```python
from build123d import *

# Parameters (mm, degrees)
SKETCH1_R           = 1.27
BOSS_EXTRUDE1_DEPTH = 0.4
SKETCH2_W           = 11.275942915
SKETCH2_H           = 6.002616378
BOSS_EXTRUDE2_DEPTH = 2.4


with BuildPart() as part:
    # Sketch1 → Boss-Extrude1 (new body)
    with BuildSketch(Plane(origin=(0, 0, 0), x_dir=(1, 0, 0), z_dir=(0, 1, 0))):
        with BuildLine():
            Line((13.97, -10.16), (-13.97, -10.16))
            ThreePointArc((-13.97, -10.16), (-15.766051224, -9.416051224), (-16.51, -7.62))
            Line((-16.51, -7.62), (-16.51, 7.62))
            ThreePointArc((-16.51, 7.62), (-15.766051224, 9.416051224), (-13.97, 10.16))
            Line((-13.97, 10.16), (13.97, 10.16))
            ThreePointArc((13.97, 10.16), (15.766051224, 9.416051224), (16.51, 7.62))
            Line((16.51, 7.62), (16.51, -7.62))
            ThreePointArc((16.51, -7.62), (15.766051224, -9.416051224), (13.97, -10.16))
        make_face()
        with Locations(Location((-13.97, 7.62, 0), (0, 0, 270))):
            Circle(SKETCH1_R, mode=Mode.SUBTRACT)
        with Locations(Location((13.97, 7.62, 0), (0, 0, 270))):
            Circle(SKETCH1_R, mode=Mode.SUBTRACT)
        with Locations(Location((13.97, -7.62, 0), (0, 0, 270))):
            Circle(SKETCH1_R, mode=Mode.SUBTRACT)
        with Locations(Location((-13.97, -7.62, 0), (0, 0, 270))):
            Circle(SKETCH1_R, mode=Mode.SUBTRACT)
    extrude(amount=BOSS_EXTRUDE1_DEPTH)

    # Sketch2 → Boss-Extrude2 (add)
    with BuildSketch(Plane(origin=(0, 0.4, 0), x_dir=(1, 0, 0), z_dir=(0, 1, 0))):
        with Locations((-5.637971457, 0)):
            Rectangle(SKETCH2_W, SKETCH2_H)
    extrude(amount=BOSS_EXTRUDE2_DEPTH)


solid = part.part
```
Part model, mm, in its own coordinate system. A direction names the side the tool comes from. Give positions to 0.01 mm unless a question says otherwise; leave off trailing zeros. Write each loop counter-clockwise with the first axis right and the second up, starting at its lowest first coordinate (ties: lowest second). Pieces come first, ordered by that corner, then holes. Notation, with made-up numbers: M 25.25,81 L 35.25,81 A13 cw 35.25,95 Z; hole C 18,27.5 d7. An arc over 180 degrees is marked long. Use CSV: the item, a comma, the result in double quotes.
Item 1: Slice it at C-C on z = 8. Write the cut outline in (x, y), plus the area to 3 significant figures.
Taken from the geometry:
outline,"M -16.48,0 L -15.18,0 L -15.18,0.4 L -16.48,0.4 Z; M -12.76,0 L 12.76,0 L 12.76,0.4 L -12.76,0.4 Z; M 15.18,0 L 16.48,0 L 16.48,0.4 L 15.18,0.4 Z"
area,"11.2 mm²"
Item 2: Pull direction X, two halves, no side cores. Call faces 4 (the face through (-12.71, 0.2, -7.79)), 5 (the face through (-15.746, 0.197, 9.436)), 6 (the face through (0, 2, 0)), 7 (the face through (0.2, 0.4, -0.1)): +X half, -X half, draft (parallel to the pull), parting line (faces both ways), or undercut.
Taken from the geometry:
face 4,"undercut"
face 5,"-X half"
face 6,"+X half"
face 7,"draft"
Item 3: Which spindle directions (+Z, -Z, +X, -X, +Y, -Y) get a long thin tool onto all of the face, cutting with end or side? Do faces 1 (the face through (-6, 2, -3.001)), 2 (the face through (-11.276, 2, 0)), 3 (the face through (-6, 2, 3.001)). Say none if no direction does.
Taken from the geometry:
face 1,"-Z, +X, -X, +Y"
face 2,"+Z, -Z, -X, +Y"
face 3,"+Z, +X, -X, +Y"
Item 4: Slice it at D-D on y = 2.3. Write the cut outline in (x, z).
Taken from the geometry:
outline,"M -11.28,-3 L 0,-3 L 0,3 L -11.28,3 Z"
Item 5: Slice it at A-A on z = 1.75. Write the cut outline in (x, y), plus the area to 3 significant figures.
Taken from the geometry:
outline,"M -16.51,0 L 16.51,0 L 16.51,0.4 L 0,0.4 L 0,2.8 L -11.28,2.8 L -11.28,0.4 L -16.51,0.4 Z"
area,"40.3 mm²"
Item 6: Drill centre lines: probe 1 along X at (y, z) = (0.1, -7.62); probe 2 along Y at (x, z) = (1, 2.25); probe 3 along Z at (x, y) = (-3, 1.5). Where is each one in solid material? Low to high.
Taken from the geometry:
probe 1,"x = -16.51 to -15.24, -12.7 to 12.7, 15.24 to 16.51"
probe 2,"y = 0 to 0.4"
probe 3,"z = -3 to 3"
Item 7: Slice it at B-B on x = -1. Write the cut outline in (y, z).
Taken from the geometry:
outline,"M 0,-10.16 L 0.4,-10.16 L 0.4,-3 L 2.8,-3 L 2.8,3 L 0.4,3 L 0.4,10.16 L 0,10.16 Z"
Item 8: Pin check, flat tips, straight feed: P1, Ø0.7, axis at x = -4.5, y = 1.5, coming from the -Z side; P2, Ø0.7, axis at y = 1.5, z = 0, coming from the -X side; P3, Ø1.5, axis at x = -13.97, z = 7.62, coming from the -Y side; P4, Ø3.5, axis at x = 13.97, z = -7.62, coming from the +Y side. Stop position of each tip, or through.
Taken from the geometry:
P1,"stops at z = -3"
P2,"stops at x = -11.28"
P3,"passes through"
P4,"stops at y = 0.4"
